```python
from build123d import *

# Parameters (mm, degrees)
F0_R      = 12
F1_DEPTH  = 2
F3_DEPTH  = 2
F4_R      = 1.5
F5_DEPTH  = 25
F6_SIZE   = 0.5
F7_R      = 6.35
F8_DEPTH  = 25
F9_R      = 1.5
F10_DEPTH = 25
F11_SIZE  = 0.5


with BuildPart() as f1:
    # F0 (on Front) → F1 (new body)
    with BuildSketch(Plane.XZ):
        with BuildLine():
            ThreePointArc((64.5, -22.5), (87, 0), (64.5, 22.5))
            Line((64.5, 22.5), (-64.5, 22.5))
            ThreePointArc((-64.5, 22.5), (-87, 0), (-64.5, -22.5))
            Line((-64.5, -22.5), (64.5, -22.5))
        make_face()
        with Locations((-64.5, 0)):
            Circle(F0_R, mode=Mode.SUBTRACT)
        with Locations((64.5, 0)):
            Circle(F0_R, mode=Mode.SUBTRACT)
    extrude(amount=F1_DEPTH)

    # F2 (on face) → F3 (join)
    with BuildSketch(Plane.XZ.offset(2)):
        Polygon((-87, -22.5), (-64.5, -22.5), (-64.5, -17.4313578755), (-70.5482587218, -14.7617282346), (-78.2682448626, -9.4630774111), (-80.8771923184, 0), (-87, 0), align=None)
    extrude(amount=-F3_DEPTH)

    # F4 (on face) → F5 (cut)
    with BuildSketch(Plane.XZ.offset(2)):
        with Locations((-53.5, 16)):
            Circle(F4_R)
        with Locations((-53.5, -16)):
            Circle(F4_R)
        with Locations((53.5, 16)):
            Circle(F4_R)
        with Locations((53.5, -16)):
            Circle(F4_R)
    extrude(amount=-F5_DEPTH, mode=Mode.SUBTRACT)

    # F6
    f6_edges = [f1.edges().sort_by_distance(p)[0] for p in [
        (-55, 0, 16),
        (-55, 0, -16),
        (52, 0, 16),
        (52, 0, -16),
    ]]
    chamfer(f6_edges, length=F6_SIZE)

    # F7 (on face) → F8 (cut)
    with BuildSketch(Plane.XZ.offset(2)):
        Circle(F7_R)
    extrude(amount=-F8_DEPTH, mode=Mode.SUBTRACT)

    # F9 (on face) → F10 (cut)
    with BuildSketch(Plane.XZ.offset(2)):
        with Locations((-11.35, 4)):
            Circle(F9_R)
        with Locations((-11.35, -4)):
            Circle(F9_R)
        with Locations((11.35, 4)):
            Circle(F9_R)
        with Locations((11.35, -4)):
            Circle(F9_R)
    extrude(amount=-F10_DEPTH, mode=Mode.SUBTRACT)

    # F11
    f11_edges = [f1.edges().sort_by_distance(p)[0] for p in [
        (-12.85, 0, 4),
        (-12.85, 0, -4),
        (9.85, 0, -4),
        (9.85, 0, 4),
    ]]
    chamfer(f11_edges, length=F11_SIZE)


solid = f1.part
```
Source: CAD feature listing. Evaluate the final solid. Frame: model axes, mm. Round coordinates to 2 decimals unless told otherwise and drop trailing zeros. Loops run counter-clockwise (first coordinate to the right, second up) from the corner with the lowest first, then second, coordinate; pieces in that order, holes last. Notation, with made-up numbers: M 47.5,-12.5 L 52.5,-12.5 A10 ccw 52.5,0.5 Z; hole C -13.5,-38.75 d3. An arc over 180 degrees is marked long. Use a Markdown table: item, result. Add a question column.
1. Pull-direction query (X, two-part tool) for faces 1 (the cylindrical face through (87, -1, 0)), 2 (the cylindrical face through (12.156, -1.26, 5.265)), 3 (the flat face through (-1, -2, -10)); classes: +X half, -X half, draft (parallel to the pull), parting line (faces both ways), or undercut.
2. Cut plane B-B, the plane y = -0.95. State how many separate pieces and enclosed holes the cut face has, and give its area (3 significant figures).
3. Cut plane D-D, the plane x = -71.5. Output: boundary loops of the cut face in (y, z), and give its area (3 significant figures).
4. Ray query, line 1 along Z through (x, y) = (-11.35, -1.15); line 2 along Z through (x, y) = (10.5, -0.75); line 3 along X through (y, z) = (-0.2, -1). Return the intervals inside material, ascending. Write a range as [from, to].
5. Contact query for flat-ended pins moving along their axis: pin 1 (8 mm diameter, centred on x = -8.5, z = -14.5, fed in from +Y); pin 2 (3.5 mm diameter, centred on x = 53.5, z = 16, fed in from +Y). Output: stop coordinate, or through.
6. Cut plane A-A, the plane x = -11.35. Output: boundary loops of the cut face in (y, z), and give its area (3 significant figures).
7. Cut plane C-C, the plane z = -16. Output: boundary loops of the cut face in (x, y).
Solution:
| question | item | result |
|---|---|---|
| 1 | face 1 | +X half |
| 1 | face 2 | undercut |
| 1 | face 3 | draft |
| 2 | separate pieces | 1 |
| 2 | enclosed holes | 11 |
| 2 | area | 6,420 mm2 |
| 3 | outline | M -2,-22.5 L 0,-22.5 L 0,-9.75 L -2,-9.75 Z; M -2,9.75 L 0,9.75 L 0,21.38 L -2,21.38 Z |
| 3 | area | 48.8 mm2 |
| 4 | line 1 | z = [-22.5, -5.5], [-2.5, 2.5], [5.5, 22.5] |
| 4 | line 2 | z = [-22.5, -5.24], [-2.76, 2.76], [5.24, 22.5] |
| 4 | line 3 | x = [-87, -76.46], [-52.54, -6.27], [6.27, 52.54], [76.46, 86.98] |
| 5 | pin 1 | stops at y = 0 |
| 5 | pin 2 | stops at y = -0.25 |
| 6 | outline | M -2,-22.5 L 0,-22.5 L 0,-6 L -0.5,-5.5 L -2,-5.5 Z; M -2,-2.5 L -0.5,-2.5 L 0,-2 L 0,2 L -0.5,2.5 L -2,2.5 Z; M -2,5.5 L -0.5,5.5 L 0,6 L 0,22.5 L -2,22.5 Z |
| 6 | area | 77.5 mm2 |
| 7 | outline | M -87,-2 L -55,-2 L -55,-0.5 L -55.5,0 L -87,0 Z; M -52,-2 L 52,-2 L 52,-0.5 L 51.5,0 L -51.5,0 L -52,-0.5 Z; M 55,-2 L 80.32,-2 L 80.32,0 L 55.5,0 L 55,-0.5 Z |
